The listing builds one solid part. Answer for the finished solid, in the listing's coordinates (mm). A direction names the side the tool comes from. Round coordinates to 2 decimals unless told otherwise and drop trailing zeros. Order: outer loops, then holes, each group sorted by start corner. A loop starts at its lowest first (then second) coordinate and runs counter-clockwise, first axis right, second up. Notation, with made-up numbers: (-18.5, 50) - (-13.5, 50) arc R14 ccw to (-13.5, 71) - close; hole circle Ø8 at (-23, -27). An arc over 180 degrees is marked (long way). Use CSV: the item, a comma, the result in double quotes. Start each with the question number.
Item 1: Straight lines are drawn through the part: line 1 along Y through (x, z) = (-9.5, 8.25); line 2 along Y through (x, z) = (-13, 3.5); line 3 along Z through (x, y) = (0.5, 2). For each, find the intervals that lie inside material, in ascending order. Write a range as [from, to].
Item 2: Determine the mould class of faces 4 (the flat face through (0, 22, 11.5)), 5 (the flat face through (-1, 22.5, 9)), 6 (the flat face through (-10.5, 22, 15)), 7 (the flat face through (13.79, 22, 9)) for opening direction X: +X half, -X half, draft (parallel to the pull), parting line (faces both ways), or undercut.
Item 3: Find section B-B, the plane z = 9. Give the vertices of the cut face in (x, y).
Item 4: Find section D-D, the plane x = -0.25. Give the vertices of the cut face in (y, z), plus the area to 3 significant figures.
Item 5: Find section A-A, the plane z = 6.5. Give the vertices of the cut face in (x, y).
Item 6: For faces 1 (the flat face through (10.5, 22, 4)), 2 (the flat face through (10.5, 22, 15)), 3 (the flat face through (0, 5, 8.5)), determine the directions among +Z, -Z, +X, -X, +Y, -Y from which every point of the face is accessible in a straight line to the end or side of a thin tool.
Item 7: Flat-ended cylindrical pins translate along their axes: P1, Ø2, axis at x = -3, y = 21, coming from the +Z side; P2, Ø1, axis at y = -4, z = 12.5, coming from the -X side; P3, Ø5.5, axis at x = 0.5, y = 5.5, coming from the -Z side; P4, Ø3, axis at y = 14.5, z = 15, coming from the +X side. Find the tip coordinate at first contact, or state that the pin passes through.
Item 8: Find section C-C, the plane y = 20. Give the vertices of the cut face in (x, z).
Autodesk Inventor part; units mm, degrees
ref_plane "Work Plane5" through (0, 0, 9.5) normal (0, 0, 1) x (1, 0, 0)
ref_plane "Work Plane4" through (-12.5, 22.5, 0) normal (0, 1, 0) x (1, 0, 0)
ref_plane "YZ Plane" through (0, 0, 0) normal (1, 0, 0) x (0, 1, 0)
ref_plane "Work Plane5" through (0, 0, 9.5) normal (0, 0, 1) x (1, 0, 0)
sketch "Sketch4" plane through (0, 0, 9.5) normal (0, 0, 1) x (1, 0, 0)
  arc A0 (-3.3085, -7.69) -> (3.0707, -6.4871) centre (-0.1029, -7.1736) ccw
  line L0 (3.0707, -6.4871) -> (3.7901, 20.5)
  line L1 (-2.7798, 20.5) -> (-3.3085, -7.69)
  line L2 (-3.8298, 20.5) -> (-2.7798, 20.5)
  line L3 (3.7901, 20.5) -> (4.8401, 20.5)
  line L4 (-11.5, 20.5) -> (-12.5, 20.5)
  line L5 (11.5, 20.5) -> (9.5, 20.5)
  line L6 (-12.5, 20.5) -> (-2.7798, 20.5)
  line L7 (3.7901, 20.5) -> (18.7901, 20.5)
  line L8 (-12.5, 20.5) -> (-12.5, 14.637)
  line L9 (-12.5, 14.637) -> (-12.5, 20.5)
  line L10 (-12.5, 14.637) -> (-14.5, 14.637)
  line L11 (-14.5, 14.637) -> (-14.5, 22.5)
  line L12 (-14.5, 22.5) -> (18.7901, 22.5)
  line L13 (18.7901, 22.5) -> (18.7901, 20.5)
  line L14 (-2.7798, 20.5) -> (3.7901, 20.5)
  point P0 (0, 0)
  point P1 (-0.3189, -10.4133)
  dimension "d34" = 15
  dimension "d36" = 2
extrude "Extrusion7" add sketch "Sketch4" along normal mid plane 2 contours L1 L14 L0 A0
extrude "Extrusion8" add sketch "Sketch4" along normal mid plane 17 contours L2 L6 L4 L8 L10 L11 L12 L13 L7 L5 L3 L14
ref_plane "Work Plane4" through (-12.5, 22.5, 0) normal (0, 1, 0) x (1, 0, 0)
sketch "Sketch5" plane through (-12.5, 22.5, 0) normal (0, 1, 0) x (1, 0, 0)
  line L0 (-2, -11.5) -> (27, -11.5)
  line L1 (27, -11.5) -> (27, -7.5)
  line L2 (27, -7.5) -> (-2, -7.5)
  line L3 (-2, -7.5) -> (-2, -11.5)
  line L4 (15.5, -9.5) -> (9.5, -9.5)
  line L5 (-2, -11.5) -> (27, -7.5) construction
  line L6 (27, -11.5) -> (-2, -7.5) construction
  line L7 (0, -1) -> (25, -1)
  line L8 (25, -1) -> (25, -7.5)
  line L9 (25, -7.5) -> (0, -7.5)
  line L10 (0, -7.5) -> (0, -1)
  line L11 (0, -9.5) -> (0, -18)
  line L12 (0, -18) -> (31.2901, -18)
  line L13 (0, -11.5) -> (25, -11.5)
  line L14 (25, -11.5) -> (25, -18)
  line L15 (25, -18) -> (0, -18)
  line L16 (0, -18) -> (0, -11.5)
  point P0 (12.5, 0)
  point P1 (12.5, -9.5)
extrude "Extrusion9" cut sketch "Sketch5" against normal through all contours L0 L14 L12 L11 | L10 L7 L8 L2
sketch "Sketch6" plane through (-14.5, 22.5, 1) normal (0, 1, 0) x (1, 0, 0)
  line L0 (2, -6.5) -> (27, -6.5)
  line L1 (2, 0) -> (4, 0)
  line L2 (4, 0) -> (4, -6.5)
  line L3 (4, -6.5) -> (2, -6.5)
  line L4 (2, -6.5) -> (2, 0)
  line L5 (27, -10.5) -> (2, -10.5)
  line L6 (2, -17) -> (4, -17)
  line L7 (4, -17) -> (4, -10.5)
  line L8 (4, -10.5) -> (2, -10.5)
  line L9 (2, -10.5) -> (2, -17)
  line L10 (27, 0) -> (25, 0)
  line L11 (25, 0) -> (25, -6.5)
  line L12 (25, -6.5) -> (27, -6.5)
  line L13 (27, -6.5) -> (27, 0)
  line L14 (27, -10.5) -> (25, -10.5)
  line L15 (25, -10.5) -> (25, -17)
  line L16 (25, -17) -> (27, -17)
  line L17 (27, -17) -> (27, -10.5)
  point P0 (14.5, 1)
  dimension "d43" = 2
  dimension "d44" = 2
  dimension "d45" = 2
  dimension "d46" = 2
extrude "Extrusion10" add sketch "Sketch6" against normal blind 2
sketch "Sketch7" plane through (18.7901, 22.5, 18) normal (0, 1, 0) x (1, 0, 0)
  line L0 (-8.2901, 0) -> (0, 0)
  line L1 (0, 17) -> (-5, 17)
  line L2 (-5, 17) -> (-5, 0)
  line L3 (-5, 0) -> (0, 0)
  line L4 (0, 0) -> (0, 17)
  point P0 (-18.7901, 18)
  dimension "d49" = 5
extrude "Extrusion11" cut sketch "Sketch7" against normal through all
properties part number "cover sepatu"
Worked out:
1,line 1,"y = [20.5, 22.5]"
1,line 2,"y = [14.64, 22.5]"
1,line 3,"z = [8.5, 10.5]"
2,face 4,"undercut"
2,face 5,"draft"
2,face 6,"undercut"
2,face 7,"+X half"
3,outline,"(-14.5, 14.64) - (-12.5, 14.64) - (-12.5, 20.5) - (-2.78, 20.5) - (-3.31, -7.69) arc R3.25 ccw (long way) to (3.07, -6.49) - (3.79, 20.5) - (13.79, 20.5) - (13.79, 22.5) - (-14.5, 22.5) - close"
4,outline,"(-10.42, 8.5) - (20.5, 8.5) - (20.5, 7.5) - (22.5, 7.5) - (22.5, 11.5) - (20.5, 11.5) - (20.5, 10.5) - (-10.42, 10.5) - close"
4,area,"69.8 mm²"
5,outline,"(-14.5, 14.64) - (-12.5, 14.64) - (-12.5, 20.5) - (-10.5, 20.5) - (-10.5, 22.5) - (-14.5, 22.5) - close; (10.5, 20.5) - (13.79, 20.5) - (13.79, 22.5) - (10.5, 22.5) - close"
6,face 1,"-Z, +Y, -Y"
6,face 2,"+Z, +Y, -Y"
6,face 3,"-Z, +X, -Y"
7,P1,"stops at z = 11.5"
7,P2,"passes through"
7,P3,"stops at z = 8.5"
7,P4,"stops at x = -12.5"
8,outline,"(-14.5, 1) - (-12.5, 1) - (-12.5, 18) - (-14.5, 18) - close; (-2.79, 8.5) - (3.78, 8.5) - (3.78, 10.5) - (-2.79, 10.5) - close"
